Input: part model. Units: mm. Frame: model coordinates. A direction names the side the tool comes from. Give positions to 0.01 mm unless a question says otherwise; leave off trailing zeros. Order: outer loops, then holes, each group sorted by start corner. A loop starts at its lowest first (then second) coordinate and runs counter-clockwise, first axis right, second up. Notation, with made-up numbers: (-10, -13) - (25, -13) arc R11 cw to (25, -6) - close; hole circle Ø9 at (59.25, -19.5). An arc over 180 degrees is marked (long way). Use a Markdown table: item, result.
from build123d import *

# Parameters (mm, degrees)
BOSS_EXTRUDE1_DEPTH = 170
CUT_EXTRUDE1_DEPTH  = 165
SKETCH5_W           = 35
SKETCH5_H           = 28
CUT_EXTRUDE3_DEPTH  = 228.794623549
SKETCH6_W           = 35
SKETCH6_H           = 28
CUT_EXTRUDE5_DEPTH  = 228.794623549
SKETCH8_W           = 35
SKETCH8_H           = 28
CUT_EXTRUDE9_DEPTH  = 228.794623549


with BuildPart() as part:
    # Sketch2 → Boss-Extrude1 (new body)
    with BuildSketch(Plane(origin=(0, 0, 0), x_dir=(0, 0, -1), z_dir=(1, 0, 0))):
        Polygon((150, 10), (150, -15), (0, -15), (0, 0), align=None)
    extrude(amount=-BOSS_EXTRUDE1_DEPTH)

    # Sketch3 → Cut-Extrude1 (cut)
    with BuildSketch(Plane.ZY.offset(170)):
        Polygon((-145, 9.666666667), (-145, -11.8), (-5, -12.6), (-5, 0.333333333), align=None)
    extrude(amount=-CUT_EXTRUDE1_DEPTH, mode=Mode.SUBTRACT)

    # Sketch5 → Cut-Extrude3 (cut, through all)
    with BuildSketch(Plane(origin=(0, -12.628159081, -0.072160909), x_dir=(1, 0, 0), z_dir=(0, 0.9999836738692104, 0.005714192422109776))):
        with Locations((-152.5, 130.93020524)):
            Rectangle(SKETCH5_W, SKETCH5_H)
    extrude(amount=-CUT_EXTRUDE3_DEPTH, mode=Mode.SUBTRACT)

    # Sketch6 → Cut-Extrude5 (cut, through all)
    with BuildSketch(Plane(origin=(0, -12.628159081, -0.072160909), x_dir=(1, 0, 0), z_dir=(0, 0.9999836738692104, 0.005714192422109776))):
        with Locations((-152.5, 74.93020524)):
            Rectangle(SKETCH6_W, SKETCH6_H)
    extrude(amount=-CUT_EXTRUDE5_DEPTH, mode=Mode.SUBTRACT)

    # Sketch8 → Cut-Extrude9 (cut, through all)
    with BuildSketch(Plane(origin=(0, -12.628159081, -0.072160909), x_dir=(1, 0, 0), z_dir=(0, 0.9999836738692104, 0.005714192422109776))):
        with Locations((-152.5, 19.0018231)):
            Rectangle(SKETCH8_W, SKETCH8_H)
    extrude(amount=-CUT_EXTRUDE9_DEPTH, mode=Mode.SUBTRACT)


solid = part.part
1. Material intervals for line 1 along Z through (x, y) = (-138.5, -13.5); line 2 along Z through (x, y) = (-58.5, -3); line 3 along Z through (x, y) = (-70, 3), sorted ascending.
Response:
| item | result |
|---|---|
| line 1 | z = -150 to -145.01, -117.01 to -89.01, -61.01 to -33.08, -5.08 to 0 |
| line 2 | z = -150 to -145, -5 to 0 |
| line 3 | z = -150 to -145 |
2. Section query B-B (y = -9). Return loops of the section in (x, z).
Response:
| item | result |
|---|---|
| outline | (-170, -150) - (0, -150) - (0, 0) - (-170, 0) - (-170, -5) - (-5, -5) - (-5, -145) - (-170, -145) - close |
3. Section query A-A (x = -151). Return loops of the section in (y, z).
Response:
| item | result |
|---|---|
| outline | (-15, -150) - (10, -150) - (9.67, -145) - (-11.8, -145) - (-15, -145.02) - close; (-15, -117.02) - (-11.96, -117) - (-12.12, -89) - (-15, -89.02) - close; (-15, -61.02) - (-12.28, -61) - (-12.44, -33.07) - (-15, -33.09) - close; (-15, -5.09) - (-12.6, -5.07) - (-12.6, -5) - (0.33, -5) - (0, 0) - (-15, 0) - close |
4. Pin query (flat end, axial travel): pin 1 (5 mm diameter, centred on y = -6.5, z = -116, fed in from -X); pin 2 (0.9 mm diameter, centred on y = -14, z = -75, fed in from -X); pin 3 (10 mm diameter, centred on x = -34.5, z = -120, fed in from +Y). Return the tip coordinate at first contact, or that it passes through.
Response:
| item | result |
|---|---|
| pin 1 | stops at x = -5 |
| pin 2 | stops at x = -135 |
| pin 3 | stops at y = -11.91 |
5. Set-up query: faces 5 (the face through (0, -5, -76)), 6 (the face through (-5, -4, -76)). Return all of +Z, -Z, +X, -X, +Y, -Y with unobstructed straight access to the full face (end or side cutting, diameter ignored); none if empty.
Response:
| item | result |
|---|---|
| face 5 | +Z, -Z, +X, +Y, -Y |
| face 6 | -X, +Y |
6. Section query D-D (z = -121.5). Return loops of the section in (x, y).
Response:
| item | result |
|---|---|
| outline | (-135, -15) - (0, -15) - (0, 8.1) - (-5, 8.1) - (-5, -11.93) - (-135, -11.93) - close |
7. Section query C-C (x = -38.5). Return loops of the section in (y, z).
Response:
| item | result |
|---|---|
| outline | (-15, -150) - (10, -150) - (9.67, -145) - (-11.8, -145) - (-12.6, -5) - (0.33, -5) - (0, 0) - (-15, 0) - close |
8. Mould query, pull axis Z, two halves, no side actions, for faces 1 (the face through (-170, -2, -148)), 2 (the face through (-3, 5, -75)), 3 (the face through (-89, -1, -145)), 4 (the face through (-89, -6, -5)). Classes: pulls with the +Z half, pulls with the -Z half, needs draft (parallel to the pull), parting line crosses it, or undercut.
Response:
| item | result |
|---|---|
| face 1 | needs draft |
| face 2 | pulls with the +Z half |
| face 3 | undercut |
| face 4 | undercut |
